Autodesk Fusion 360 part; units mm, degrees
sketch "Skizze1" plane through (0, 0, 0) normal (0, 0, 1) x (1, 0, 0)
  line L0 (0, 0) -> (52.6, 0)
  line L1 (52.6, 0) -> (52.6, 25.6)
  line L2 (52.6, 25.6) -> (0, 25.6)
  line L3 (0, 25.6) -> (0, 0)
  line L4 (0, 0) -> (50.8, 0)
  line L5 (3.2, 3.2) -> (49.4, 3.2)
  line L6 (49.4, 3.2) -> (49.4, 22.4)
  line L7 (49.4, 22.4) -> (3.2, 22.4)
  line L8 (3.2, 22.4) -> (3.2, 3.2)
  line L9 (1.6, 24) -> (51, 24)
  line L10 (51, 24) -> (51, 1.6)
  line L11 (51, 1.6) -> (1.6, 1.6)
  line L12 (1.6, 1.6) -> (1.6, 24)
  circle A0 centre (8.2, 22.4) radius 1
  circle A1 centre (44.1, 22.4) radius 1
  circle A2 centre (44.1, 3.2) radius 1
  circle A3 centre (8.2, 3.2) radius 1
  dimension "d2" = 46.2
  dimension "d3" = 19.2
  dimension "d4" = 1.6
  dimension "d6" = 1.6
  dimension "d7" = 1.6
  dimension "d8" = 1.6
  dimension "d13" = 1.6
  dimension "d14" = 1.6
  dimension "d15" = 1.6
  dimension "d16" = 1.6
  dimension "d28" = 2
  dimension "d29" = 2
  dimension "d30" = 2
  dimension "d31" = 2
  dimension "d32" = 5.3
  dimension "d33" = 5.3
  dimension "d34" = 5
  dimension "d35" = 5
extrude "Extrusion1" add sketch "Skizze1" along normal blind 1.6 contours L0 L1 L2 L3 L4 | L5 L6 L7 L8 A0 A1 A2 A3 | L5 A2 | L5 A2 | L5 A3 | L5 A3 | L7 A1 | L7 A1 | L7 A0 | L7 A0 | L9 L10 L11 L12
extrude "Extrusion2" add sketch "Skizze1" along normal blind 7 contours L5 A2 | L5 A3 | L7 A1 | L7 A0 | L9 L10 L11 L12 picked at (44.1779, 2.8253) picked at (7.9246, 2.9129) picked at (44.3078, 22.76) picked at (8.5222, 22.5479)
ref_plane "Arbeitsebene1" through (1.6, 12.8, 4.3) normal (-1, 0, 0) x (0, -1, 0)
sketch "Skizze2" plane through (1.6, 0, 0) normal (-1, 0, 0) x (0, -1, 0)
  line L0 (-17.3, 7) -> (-8.3, 7)
  line L1 (-8.3, 7) -> (-8.3, 3.7)
  line L2 (-8.8, 3.2) -> (-16.8, 3.2)
  line L3 (-17.3, 3.7) -> (-17.3, 7)
  line L4 (-24, 7) -> (-1.6, 7)
  line L5 (-25.6, 1.6) -> (0, 1.6)
  arc A0 (-17.3, 3.7) -> (-16.8, 3.2) centre (-16.8, 3.7) ccw
  arc A1 (-8.8, 3.2) -> (-8.3, 3.7) centre (-8.8, 3.7) ccw
  dimension "d22" = 1.6
  dimension "d23" = 9
  dimension "d24" = 0.5
  dimension "d25" = 0.5
extrude "Extrusion3" cut sketch "Skizze2" against normal blind 1.6
extrude "Extrusion4" add sketch "Skizze1" along normal blind 3.2 contours L5 A2 | L5 A3 | L7 A1 | L7 A0 picked at (44.0258, 3.6243) picked at (8.0222, 3.8816) picked at (44.3444, 22.0739) picked at (7.9673, 21.807)
equation "d19 = 1.6 mm + 4.9 mm + 0.5 mm"
Part model, mm, in its own coordinate system. A direction names the side the tool comes from. Coordinates: 2 decimals unless noted, no trailing zeros. Write each loop counter-clockwise with the first axis right and the second up, starting at its lowest first coordinate (ties: lowest second). Pieces come first, ordered by that corner, then holes. Notation, with made-up numbers: M 76,-14 L 82,-14 A21 ccw 82,15 Z; hole C 56,-25.5 d4. An arc over 180 degrees is marked long. Return JSON: item names as keys, results as strings.
1. Flat gauge pins, fed straight in: pin 1 Ø3 at (y, z) = (12, 4) entering from -X; pin 2 Ø2 at (x, z) = (18, 3) entering from -Y; pin 3 Ø1.1 at (x, y) = (44.5, 4) entering from +Z. Where does each tip first touch, or does it go through?
Determined:
{"pin 1": "x = 1.6", "pin 2": "y = 1.6", "pin 3": "z = 3.2"}
2. Saw through at C-C, the plane x = 8.2. Write the cut outline in (y, z).
Determined:
{"outline": "M 0,0 L 25.6,0 L 25.6,1.6 L 24,1.6 L 24,7 L 22.4,7 L 22.4,3.2 L 21.4,3.2 L 21.4,1.6 L 4.2,1.6 L 4.2,3.2 L 3.2,3.2 L 3.2,7 L 1.6,7 L 1.6,1.6 L 0,1.6 Z"}
3. Saw through at A-A, the plane x = 28. Write the cut outline in (y, z), then the cut area to 3 significant figures.
Determined:
{"outline": "M 0,0 L 25.6,0 L 25.6,1.6 L 24,1.6 L 24,7 L 22.4,7 L 22.4,1.6 L 3.2,1.6 L 3.2,7 L 1.6,7 L 1.6,1.6 L 0,1.6 Z", "area": "58.2 mm²"}
4. Saw through at B-B, the plane y = 20. Write the cut outline in (x, z).
Determined:
{"outline": "M 0,0 L 52.6,0 L 52.6,1.6 L 51,1.6 L 51,7 L 49.4,7 L 49.4,1.6 L 3.2,1.6 L 3.2,7 L 1.6,7 L 1.6,1.6 L 0,1.6 Z"}
5. 3-axis set-ups, long thin cutter, end or side, ignore diameter. For faces 1 (the face through (26, 24, 4)), 2 (the face through (8, 22, 3.2)), 3 (the face through (1.6, 13, 3)), 4 (the face through (2, 8.3, 5)): which of +Z, -Z, +X, -X, +Y, -Y reach the whole face in a straight line?
Determined:
{"face 1": "+Z, +X, -X, +Y", "face 2": "+Z", "face 3": "+Z, -X, +Y, -Y", "face 4": "+Z, -X"}
6. Probe L1, parallel to Y at x = 32.5, z = 5; L2, parallel to X at y = 12, z = 2.5; L3, parallel to Z at x = 14, y = 21.5. List the from-to ranges inside material, lowest first.
Determined:
{"L1": "1.6 to 3.2, 22.4 to 24", "L2": "1.6 to 3.2, 49.4 to 51", "L3": "0 to 1.6"}
7. Pull direction Y, two halves, no side cores. Call faces 5 (the face through (26, 13, 0)), 6 (the face through (27, 25.6, 1)), 7 (the face through (2, 13, 3.2)), 8 (the face through (27, 1.6, 4)): pulls with the +Y half, pulls with the -Y half, needs draft (parallel to the pull), parting line crosses it, or undercut.
Determined:
{"face 5": "needs draft", "face 6": "pulls with the +Y half", "face 7": "undercut", "face 8": "pulls with the -Y half"}
